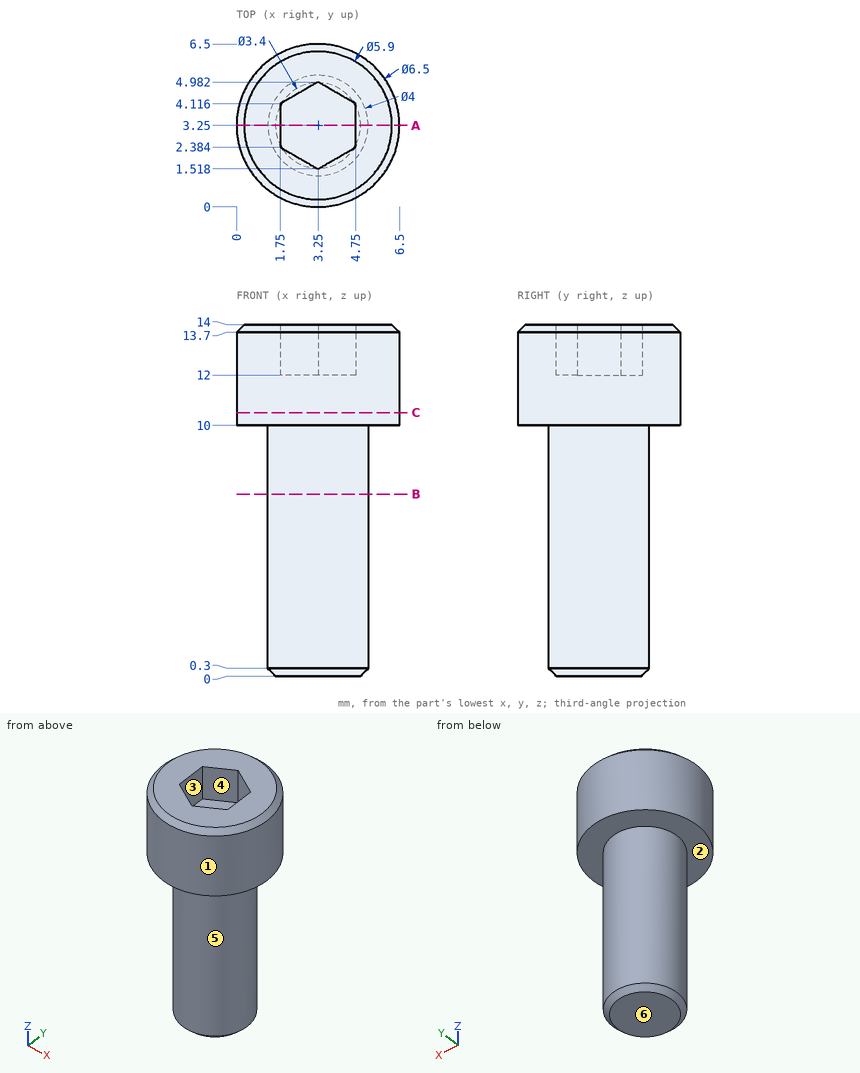
Design review of the part shown in the three views and the two pictorial views. Dimensions are in mm from the part's minimum x, y and z. A direction names the side the tool comes from. Round coordinates to 2 decimals unless told otherwise and drop trailing zeros. Write each loop counter-clockwise with the first axis right and the second up, starting at its lowest first coordinate (ties: lowest second). Pieces come first, ordered by that corner, then holes. Notation, with made-up numbers: (-2.75, 38.25) -> (20.25, 38.25) arc R27 cw to (20.25, 75.25) -> close; hole circle Ø1 at (65.5, -11.5). An arc over 180 degrees is marked (long way). Write item = value, one per line. Start each with the question number.
1) Wall thickness on probe 1 along Z at (x, y) = (3.5, 0.5); probe 2 along X at (y, z) = (3, 13.25); probe 3 along Z at (x, y) = (3.25, 2.5): over which ranges is each line inside the solid? List them lowest first. Write a range as from..to.
2) Mouldability with a two-part tool opening along X and no side actions: class the marked faces 4, 5 and 6 as +X half, -X half, draft (parallel to the pull), parting line (faces both ways), or undercut.
3) Tool access review of the marked faces 1, 2 and 3: name each direction out of +Z, -Z, +X, -X, +Y, -Y from which nothing blocks a thin tool from reaching the whole face with its end or side.
4) Take a section at B-B, the plane z = 7.25. State the section outline as (x, y) points.
5) Take a section at A-A, the plane y = 3.25. State the section outline as (x, z) points.
6) Clearance check with flat-ended pins moving along their axes: pin 1 (3 mm diameter, centred on y = 2.5, z = 4, fed in from -X); pin 2 (1 mm diameter, centred on x = 3.5, y = 3.5, fed in from +Z); pin 3 (1.5 mm diameter, centred on x = 1.5, z = 3.5, fed in from -Y). State where each tip first meets the part, or that it passes through.
7) Take a section at C-C, the plane z = 10.5. State the section outline as (x, y) points.
Results list:
q1.probe_1 = 10..14
q1.probe_2 = 0.01..1.75, 4.75..6.49
q1.probe_3 = 0..12
q2.face_4 = undercut
q2.face_5 = parting line
q2.face_6 = draft
q3.face_1 = +Z, -Z
q3.face_2 = -Z
q3.face_3 = +Z
q4.outline = circle Ø4 at (3.25, 3.25)
q5.outline = (0, 10) -> (1.25, 10) -> (1.25, 0.3) -> (1.55, 0) -> (4.95, 0) -> (5.25, 0.3) -> (5.25, 10) -> (6.5, 10) -> (6.5, 13.7) -> (6.2, 14) -> (4.75, 14) -> (4.75, 12) -> (1.75, 12) -> (1.75, 14) -> (0.3, 14) -> (0, 13.7) -> close
q6.pin_1 = 1.25
q6.pin_2 = 12
q6.pin_3 = 1.52
q7.outline = circle Ø6.5 at (3.25, 3.25)
